Could you check a few things on this drawing? It's one solid part, dimensions in mm from its lowest x, y, z. Give positions to 0.01 mm unless a question says otherwise; leave off trailing zeros. Order: outer loops, then holes, each group sorted by start corner. A loop starts at its lowest first (then second) coordinate and runs counter-clockwise, first axis right, second up.
Item 1: I want a section at C-C, the plane y = 226.5. Write out the boundary of the cut face in (x, z).
Item 2: I want a section at D-D, the plane x = 322.5. Write out the boundary of the cut face in (y, z) (1 decimal).
Item 3: If I drill on line 1 along X through (y, z) = (189.5, 3) (1 decimal); line 2 along X through (y, z) = (116, 8.5) (1 decimal); line 3 along Y through (x, z) = (359, 6) (1 decimal), over which ranges is the centre line in solid material (lowest first)?
Item 4: I'm going to push flat-ended pins straight in: pin 1 Ø10 at (y, z) = (225.5, 9.5) entering from -X; pin 2 Ø7.5 at (y, z) = (145, 16) entering from +X; pin 3 Ø5 at (y, z) = (52.5, 3.5) entering from +X. Where does each tip first touch, or does it pass through?
Item 5: I want a section at A-A, the plane z = 18.5. Write out the boundary of the cut face in (x, y) (1 decimal).
Item 6: I want a section at B-B, the plane x = 75. Write out the boundary of the cut face in (y, z).
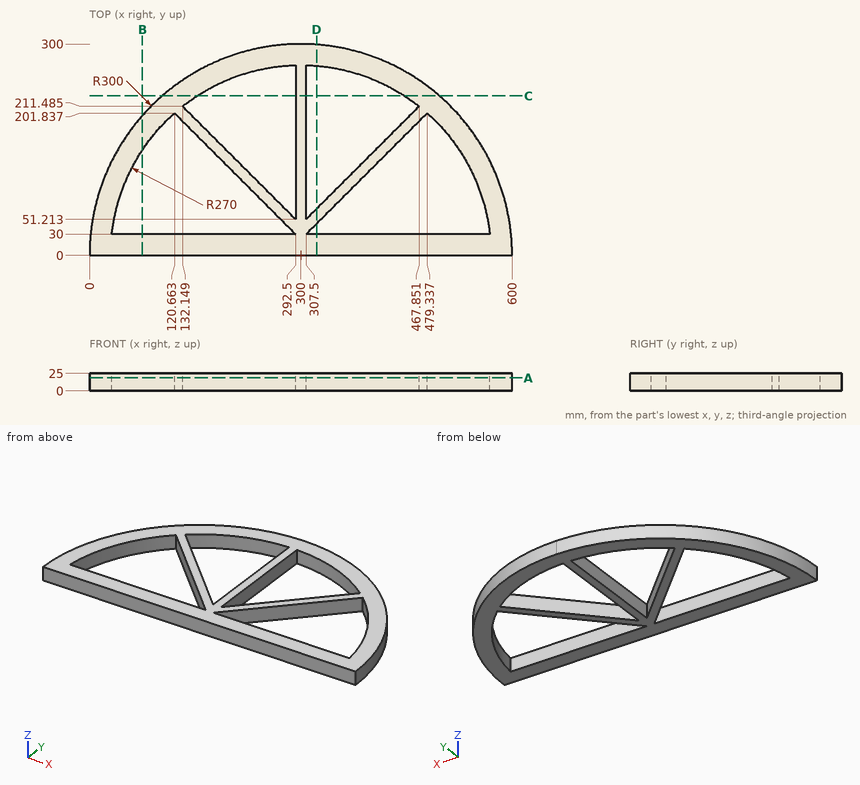
Results list:
1. outline: (103.28, 0) - (153.04, 0) - (153.04, 25) - (103.28, 25) - close; (292.5, 0) - (307.5, 0) - (307.5, 25) - (292.5, 25) - close; (446.96, 0) - (496.72, 0) - (496.72, 25) - (446.96, 25) - close
2. outline: (0, 0) - (30, 0) - (30, 25) - (0, 25) - close; (45, 0) - (66.2, 0) - (66.2, 25) - (45, 25) - close; (269.1, 0) - (299.2, 0) - (299.2, 25) - (269.1, 25) - close
3. line 1: x = 67.4 to 107.7, 133 to 154.1, 292.5 to 307.5, 445.9 to 467, 492.3 to 532.6
3. line 2: x = 23.3 to 56.2, 206.5 to 227.7, 292.5 to 307.5, 372.3 to 393.5, 543.8 to 576.7
3. line 3: y = 0 to 30, 81.5 to 102.7, 263.5 to 294.1
4. pin 1: stops at x = 96.58
4. pin 2: stops at x = 564.67
4. pin 3: stops at x = 595.8
5. outline: (0, 0) - (600, 0) arc R300 ccw to (300, 300) arc R300 ccw to start; hole (31.7, 30) - (292.5, 30) - (120.7, 201.8) arc R270 ccw to start; hole (132.1, 211.5) - (292.5, 51.2) - (292.5, 269.9) arc R270 ccw to start; hole (307.5, 30) - (568.3, 30) arc R270 ccw to (479.3, 201.8) - close; hole (307.5, 51.2) - (467.9, 211.5) arc R270 ccw to (307.5, 269.9) - close
6. outline: (0, 0) - (30, 0) - (30, 25) - (0, 25) - close; (149.25, 0) - (198.43, 0) - (198.43, 25) - (149.25, 25) - close
